For this review, take the finished solid that the model builds, in its own axes (mm). Give positions to 0.01 mm unless a question says otherwise; leave off trailing zeros. Loops run counter-clockwise (first coordinate to the right, second up) from the corner with the lowest first, then second, coordinate; pieces in that order, holes last. Notation, with made-up numbers: (-25.5, 56.5) -> (18.5, 56.5) arc R30 ccw to (18.5, 93.5) -> close; hole circle Ø3 at (-13, -38). An arc over 180 degrees is marked (long way). Answer as CSV lines item,"result". Start each with the question number.
Item 1: Add section A-A on x = 5. State the section outline as (y, z) points, plus the area to 3 significant figures.
Item 2: Clearance check with flat-ended pins moving along their axes: P1, Ø8, axis at x = 8, y = -192.5, coming from the -Z side; P2, Ø1, axis at x = -7.5, y = -545.5, coming from the +Z side; P3, Ø5, axis at y = -32, z = 0, coming from the +X side; P4, Ø10, axis at x = 10, y = -130, coming from the -Z side. State where each tip first meets the part, or that it passes through.
Item 3: For L1, parallel to Z at x = -1.25, y = -32; L2, parallel to Z at x = 0.25, y = -32; L3, parallel to Z at x = 1.25, y = -509.5, list the stretches that pass through material, from the lowest coordinate up. Write a range as from..to.
Item 4: Add section B-B on y = -628.5. State the section outline as (x, z) points, plus the area to 3 significant figures.
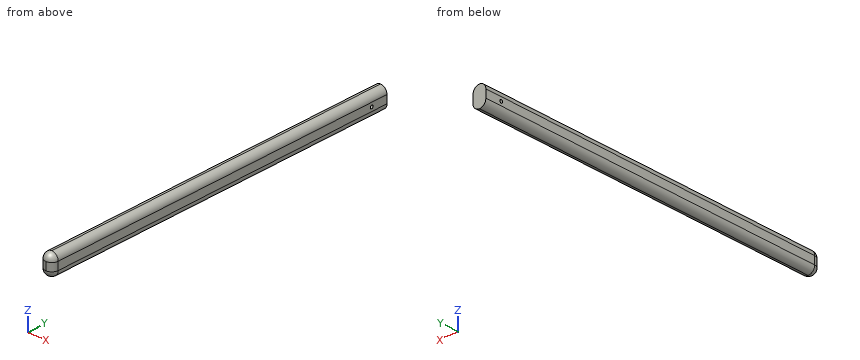
```python
from build123d import *

# Parameters (mm, degrees)
F1_DEPTH    = 700
F2_T1_DEPTH = 15
F2_T4_ANGLE = 180
F2_T6_ANGLE = 180
F3_R        = 3
F4_DEPTH    = 25.001


# Not quite as in the source:
# - a fillet or chamfer that OpenCascade refuses, or shapes differently, is made with other operations: its cross-section is extruded or revolved along the edge and cut away or added


with BuildPart() as f1:
    # F0 (on Front) → F1 (new body)
    with BuildSketch(Plane.XZ):
        with BuildLine():
            Line((12.5, -7.5), (12.5, 7.5))
            ThreePointArc((12.5, 7.5), (8.8388347648, 16.3388347648), (0, 20))
            ThreePointArc((0, 20), (-8.8388347648, 16.3388347648), (-12.5, 7.5))
            Line((-12.5, 7.5), (-12.5, -7.5))
            ThreePointArc((-12.5, -7.5), (-8.8388347648, -16.3388347648), (0, -20))
            ThreePointArc((0, -20), (8.8388347648, -16.3388347648), (12.5, -7.5))
        make_face()
    extrude(amount=F1_DEPTH)

    # F2: fillet of radius 12.5 on 4 edges, made by hand

    # F2_s2 → F2_t1 (cut)
    with BuildSketch(Plane.XY.offset(-7.5)):
        with BuildLine():
            ThreePointArc((12.5, -687.5), (8.8388347648, -696.3388347648), (0, -700))
            Line((0, -700), (12.5, -700))
            Line((12.5, -700), (12.5, -687.5))
        make_face()
        with BuildLine():
            ThreePointArc((0, -700), (-8.8388347648, -696.3388347648), (-12.5, -687.5))
            Line((-12.5, -687.5), (-12.5, -700))
            Line((-12.5, -700), (0, -700))
        make_face()
    extrude(amount=F2_T1_DEPTH, mode=Mode.SUBTRACT)

    # F2_s3 → F2_t4 (revolve, cut)
    with BuildSketch(Plane.XY.offset(-7.5)):
        with BuildLine():
            ThreePointArc((0, -700), (8.8388347648, -696.3388347648), (12.5, -687.5))
            Line((12.5, -687.5), (12.5, -700))
            Line((12.5, -700), (0, -700))
        make_face()
    revolve(axis=Axis((0, -700, -7.5), (0, 1, 0)), revolution_arc=F2_T4_ANGLE, mode=Mode.SUBTRACT)

    # F2_s5 → F2_t6 (revolve, cut)
    with BuildSketch(Plane.XY.offset(7.5)):
        with BuildLine():
            ThreePointArc((0, -700), (-8.8388347648, -696.3388347648), (-12.5, -687.5))
            Line((-12.5, -687.5), (-12.5, -700))
            Line((-12.5, -700), (0, -700))
        make_face()
    revolve(axis=Axis((0, -700, 7.5), (0, 1, 0)), revolution_arc=F2_T6_ANGLE, mode=Mode.SUBTRACT)

    # F3 (on face) → F4 (cut, through all)
    with BuildSketch(Plane(origin=(-12.5, 0, 0), x_dir=(0, -1, 0), z_dir=(-1, 0, 0))):
        with Locations((32, 0)):
            Circle(F3_R)
    extrude(amount=-F4_DEPTH, mode=Mode.SUBTRACT)


solid = f1.part
```
Computed values:
1,outline,"(-698.96, -7.5) arc R11.46 ccw to (-687.5, -18.96) -> (0, -18.96) -> (0, 18.96) -> (-687.5, 18.96) arc R11.46 ccw to (-698.96, 7.5) -> close; hole circle Ø6 at (-32, 0)"
1,area,"26,400 mm²"
2,P1,"z = -19.34"
2,P2,"z = 17.86"
2,P3,"through"
2,P4,"z = -18.96"
3,L1,"-19.94..-3, 3..19.94"
3,L2,"-20..-3, 3..20"
3,L3,"-19.94..19.94"
4,outline,"(-12.5, -7.5) arc R12.5 ccw to (12.5, -7.5) -> (12.5, 7.5) arc R12.5 ccw to (-12.5, 7.5) -> close"
4,area,"866 mm²"
